The model under review builds one solid part; all positions refer to its coordinate system, in mm. A direction names the side the tool comes from. Round coordinates to 2 decimals unless told otherwise and drop trailing zeros. Write each loop counter-clockwise with the first axis right and the second up, starting at its lowest first coordinate (ties: lowest second). Pieces come first, ordered by that corner, then holes. Notation, with made-up numbers: (69.25, -19) - (97.25, -19) arc R22 ccw to (97.25, 18) - close; hole circle Ø11 at (25.25, -8). An arc over 180 degrees is marked (long way). Use one line per item in the form item = value.
from build123d import *

# Parameters (mm, degrees)
SKETCH_1_W          = 210
SKETCH_1_H          = 35
EXTRUDE_1_DEPTH     = 5
SKETCH_2_W          = 30
SKETCH_2_H          = 5
EXTRUDE_2_DEPTH     = 20
SKETCH_3_R          = 1.65
CUT_EXTRUDE_1_DEPTH = 10
FILLET_1_R          = 3
CHAMFER_1_SIZE      = 3


with BuildPart() as part:
    # 草图1 → 凸台-拉伸1 (new body)
    with BuildSketch(Plane.XY):
        with Locations((105, 17.5)):
            Rectangle(SKETCH_1_W, SKETCH_1_H)
    extrude(amount=EXTRUDE_1_DEPTH)

    # 草图2 → 凸台-拉伸2 (add)
    with BuildSketch(Plane.XY.offset(5)):
        with Locations((55, 32.5)):
            Rectangle(SKETCH_2_W, SKETCH_2_H)
        with Locations((155, 32.5)):
            Rectangle(SKETCH_2_W, SKETCH_2_H)
    extrude(amount=EXTRUDE_2_DEPTH)

    # 草图3 → 切除-拉伸1 (cut)
    with BuildSketch(Plane(origin=(0, 35, 0), x_dir=(1, 0, 0), z_dir=(0, 1, 0))):
        with Locations(Location((160, -17, 0), (0, 0, 270))):
            Circle(SKETCH_3_R)
        with Locations(Location((150, -17, 0), (0, 0, 270))):
            Circle(SKETCH_3_R)
        with Locations(Location((60, -17, 0), (0, 0, 270))):
            Circle(SKETCH_3_R)
        with Locations(Location((50, -17, 0), (0, 0, 270))):
            Circle(SKETCH_3_R)
    extrude(amount=-CUT_EXTRUDE_1_DEPTH, mode=Mode.SUBTRACT)

    # 圆角1
    fillet_1_edges = [part.edges().sort_by_distance(p)[0] for p in [
        (40, 32.5, 25),
        (70, 32.5, 25),
        (140, 32.5, 25),
        (170, 32.5, 25),
    ]]
    fillet(fillet_1_edges, radius=FILLET_1_R)

    # 倒角1
    chamfer_1_edges = [part.edges().sort_by_distance(p)[0] for p in [
        (0, 35, 2.5),
        (210, 35, 2.5),
        (210, 0, 2.5),
        (0, 0, 2.5),
    ]]
    chamfer(chamfer_1_edges, length=CHAMFER_1_SIZE)


solid = part.part
(1) Add section A-A on z = 10. Write out the cut boundary in (x, y), then the cut area to 3 significant figures.
Geometry results:
outline = (40, 30) - (70, 30) - (70, 35) - (40, 35) - close; (140, 30) - (170, 30) - (170, 35) - (140, 35) - close
area = 300 mm2
(2) Add section B-B on y = 18. Write out the cut boundary in (x, z).
Geometry results:
outline = (0, 0) - (210, 0) - (210, 5) - (0, 5) - close
(3) To check wall thickness, follow L1, parallel to X at y = 33.3, z = 17; L2, parallel to Z at x = 160, y = 33.5; L3, parallel to Z at x = 12, y = 10.5. State the ranges of each line that lie inside material, in increasing order.
Geometry results:
L1 = 40 to 48.35, 51.65 to 58.35, 61.65 to 70, 140 to 148.35, 151.65 to 158.35, 161.65 to 170
L2 = 0 to 15.35, 18.65 to 25
L3 = 0 to 5
(4) The part is to be moulded in two halves that separate along Z. For faces 4 (the flat face through (170, 32, 13)), 5 (the cylindrical face through (148.536, 32.535, 17.761)), 6 (the flat face through (155, 33, 25)), say which applies: +Z half, -Z half, draft (parallel to the pull), parting line (faces both ways), or undercut.
Geometry results:
face_4 = draft
face_5 = undercut
face_6 = +Z half
(5) Add section C-C on x = 174. Write out the cut boundary in (y, z), then the cut area to 3 significant figures.
Geometry results:
outline = (0, 0) - (35, 0) - (35, 5) - (0, 5) - close
area = 175 mm2
(6) Machinability: for faces 1 (the flat face through (40, 32, 13)), 2 (the flat face through (140, 32, 13)), 3 (the flat face through (55, 30, 15)), which of the approach directions +Z, -Z, +X, -X, +Y, -Y give a long, thin tool a straight path to every point of the face, cutting with its end or side? Answer none if there is none.
Geometry results:
face_1 = +Z, -X, +Y, -Y
face_2 = +Z, +Y, -Y
face_3 = +Z, +X, -X, -Y
(7) Insertion check: P1, Ø17.5, axis at x = 103.5, y = 13, coming from the +Z side; P2, Ø12, axis at x = 82.5, z = 9.5, coming from the +Y side; P3, Ø2.5, axis at y = 31.5, z = 12.5, coming from the +X side; P4, Ø4, axis at y = 31.5, z = 10, coming from the -X side. Each pin has a flat end and moves straight along its axis. Give the tip position at first contact, or say it passes through.
Geometry results:
P1 = 5
P2 = 35
P3 = 170
P4 = 40
